from build123d import *

# Parameters (mm, degrees)
SKETCH1_R           = 1.778
BOSS_EXTRUDE1_DEPTH = 6.096
FILLET1_R           = 2.54
SKETCH2_R           = 2.4003
BOSS_EXTRUDE2_DEPTH = 13.97
CHAMFER1_SIZE       = 6.35
CHAMFER1_SIZE_2     = 0.667411894


with BuildPart() as part:
    # Sketch1 → Boss-Extrude1 (new, symmetric)
    with BuildSketch(Plane(origin=(0, 0, 0), x_dir=(1, 0, 0), z_dir=(0, 1, 0))):
        with BuildLine():
            Line((-10.16, 6.223), (-10.16, 13.716))
            Line((-10.16, 13.716), (10.16, 13.716))
            Line((10.16, 13.716), (10.16, 6.223))
            ThreePointArc((10.16, 6.223), (13.335, 3.048), (10.16, -0.127))
            Line((10.16, -0.127), (10.16, -13.716))
            Line((10.16, -13.716), (-10.16, -13.716))
            Line((-10.16, -13.716), (-10.16, -0.127))
            ThreePointArc((-10.16, -0.127), (-13.335, 3.048), (-10.16, 6.223))
        make_face()
        with Locations(Location((-10.16, 3.048, 0), (0, 0, 90))):
            Circle(SKETCH1_R, mode=Mode.SUBTRACT)
        with Locations(Location((10.16, 3.048, 0), (0, 0, 90))):
            Circle(SKETCH1_R, mode=Mode.SUBTRACT)
    extrude(amount=BOSS_EXTRUDE1_DEPTH, both=True)

    # Fillet1
    fillet1_edges = [part.edges().sort_by_distance(p)[0] for p in [
        (10.16, 0, -6.223),
        (10.16, 0, 0.127),
        (10.16, 0, 13.716),
        (-10.16, 0, 13.716),
        (-10.16, 0, 0.127),
        (-10.16, 0, -6.223),
        (-10.16, 0, -13.716),
        (10.16, 0, -13.716),
    ]]
    fillet(fillet1_edges, radius=FILLET1_R)

    # Sketch2 → Boss-Extrude2 (add)
    with BuildSketch(Plane(origin=(0, 6.096, 0), x_dir=(1, 0, 0), z_dir=(0, 1, 0))):
        with Locations(Location((0, 8.382, 0), (0, 0, 270))):
            Circle(SKETCH2_R)
        with Locations(Location((0, -2.286, 0), (0, 0, 270))):
            Circle(SKETCH2_R)
    extrude(amount=BOSS_EXTRUDE2_DEPTH)

    # Chamfer1
    # the kernel refuses this chamfer: 6.35, 0.667411894 mm, written as the material it adds along each edge
    with BuildSketch(Plane(origin=(0, 6.096, -8.382), x_dir=(0, 0, 1), z_dir=(-1, 0, 0))) as chamfer1_piece_1_section:
        Polygon((2.4003 + CHAMFER1_SIZE, 0), (2.4003, CHAMFER1_SIZE_2), (2.4003, 0), align=None)
    chamfer1_piece_1 = revolve(axis=Axis((0, 6.096, -8.382), (0, 1, 0)), mode=Mode.PRIVATE)
    chamfer1_piece_1 = split(chamfer1_piece_1, bisect_by=Plane(origin=(6.803322578, 6.146034246, -13.716), z_dir=(0, 0, 1)), keep=Keep.TOP, mode=Mode.PRIVATE)
    add(chamfer1_piece_1)
    with BuildSketch(Plane(origin=(0, 6.096, 2.286), x_dir=(0, 0, 1), z_dir=(-1, 0, 0))) as chamfer1_piece_2:
        Polygon((2.4003 + CHAMFER1_SIZE, 0), (2.4003, CHAMFER1_SIZE_2), (2.4003, 0), align=None)
    revolve(axis=Axis((0, 6.096, 2.286), (0, 1, 0)))
    # the kernel refuses this chamfer: 6.35, 0.667411894 mm, written as the material it takes off along each edge
    with BuildSketch(Plane(origin=(0, 20.066, -8.382), x_dir=(0, 0, 1), z_dir=(-1, 0, 0))) as chamfer1_2_piece_1:
        Polygon((2.4003, -CHAMFER1_SIZE), (2.4003 - CHAMFER1_SIZE_2, 0), (2.4003, 0), align=None)
    revolve(axis=Axis((0, 20.066, -8.382), (0, 1, 0)), mode=Mode.SUBTRACT)
    with BuildSketch(Plane(origin=(0, 20.066, 2.286), x_dir=(0, 0, 1), z_dir=(-1, 0, 0))) as chamfer1_2_piece_2:
        Polygon((2.4003, -CHAMFER1_SIZE), (2.4003 - CHAMFER1_SIZE_2, 0), (2.4003, 0), align=None)
    revolve(axis=Axis((0, 20.066, 2.286), (0, 1, 0)), mode=Mode.SUBTRACT)


solid = part.part
Work out the finished part from the listing and answer in its coordinate system (mm). A direction names the side the tool comes from. Give positions to 0.01 mm unless a question says otherwise; leave off trailing zeros. Order: outer loops, then holes, each group sorted by start corner. A loop starts at its lowest first (then second) coordinate and runs counter-clockwise, first axis right, second up. Notation, with made-up numbers: (70, 85.25) -> (99, 85.25) arc R33 cw to (99, 123.25) -> close; hole circle Ø2 at (75.5, 16). An arc over 180 degrees is marked (long way). One line per item, written item: value.
Item 1: Find section C-C, the plane x = 0. Give the vertices of the cut face in (y, z), plus the area to 3 significant figures.
Answer sheet:
outline: (-6.1, -13.72) -> (6.46, -13.72) -> (6.76, -10.78) -> (13.72, -10.78) -> (20.07, -10.11) -> (20.07, -6.65) -> (13.72, -5.98) -> (6.76, -5.98) -> (6.46, -3.05) -> (6.76, -0.11) -> (13.72, -0.11) -> (20.07, 0.55) -> (20.07, 4.02) -> (13.72, 4.69) -> (6.76, 4.69) -> (6.1, 11.04) -> (6.1, 13.72) -> (-6.1, 13.72) -> close
area: 467 mm²
Item 2: Find section D-D, the plane y = 7.5. Give the vertices of the cut face in (x, z), plus the area to 3 significant figures.
Answer sheet:
outline: circle Ø4.8 at (0, -8.38); circle Ø4.8 at (0, 2.29)
area: 36.2 mm²
Item 3: Find section A-A, the plane y = -0.75. Give the vertices of the cut face in (x, z) (3 decimals).
Answer sheet:
outline: (-11.571, -5.892) arc R2.54 cw to (-10.16, -8.168) -> (-10.16, -11.176) arc R2.54 ccw to (-7.62, -13.716) -> (7.62, -13.716) arc R2.54 ccw to (10.16, -11.176) -> (10.16, -8.168) arc R2.54 cw to (11.571, -5.892) arc R3.175 ccw to (11.571, -0.204) arc R2.54 cw to (10.16, 2.072) -> (10.16, 11.176) arc R2.54 ccw to (7.62, 13.716) -> (-7.62, 13.716) arc R2.54 ccw to (-10.16, 11.176) -> (-10.16, 2.072) arc R2.54 cw to (-11.571, -0.204) arc R3.175 ccw to start; hole circle Ø3.556 at (-10.16, -3.048); hole circle Ø3.556 at (10.16, -3.048)
Item 4: Straight lines are drawn through the part: probe 1 along X at (y, z) = (5, -2); probe 2 along X at (y, z) = (-1.75, 4.5); probe 3 along Z at (x, y) = (-1.5, 12). For each, find the intervals that lie inside material, in ascending order.
Answer sheet:
probe 1: -13.16 to -11.6, -8.72 to 8.72, 11.6 to 13.16
probe 2: -10.16 to 10.16
probe 3: -10.26 to -6.51, 0.41 to 4.16
Item 5: Find section B-B, the plane x = -9.75. Give the vertices of the cut face in (y, z), plus the area to 3 significant figures.
Answer sheet:
outline: (-6.1, -12.56) -> (6.1, -12.56) -> (6.1, -4.78) -> (-6.1, -4.78) -> close; (-6.1, -1.32) -> (6.1, -1.32) -> (6.1, 12.56) -> (-6.1, 12.56) -> close
area: 264 mm²
Item 6: A tool of negligible diameter and unlimited length cuts with its end or side. For faces 1 (the flat face through (10.16, 0, 7)), 2 (the cylindrical face through (0.721, 10.191, 4.575)), 3 (the flat face through (0, 0, -13.716)), from which of +Z, -Z, +X, -X, +Y, -Y can it reach the whole face along a straight path? Write none if from no direction.
Answer sheet:
face 1: +Z, +X, +Y, -Y
face 2: +Y
face 3: -Z, +X, -X, +Y, -Y
Item 7: Determine the mould class of faces 4 (the cylindrical face through (0.11, 10.19, -10.78)), 5 (the conical face through (-0.79, 16.94, -6.48)), 6 (the cylindrical face through (-13.335, 0.085, -2.999)), 7 (the flat face through (-10.16, 0, 7)) for opening direction Z: released by +Z, released by -Z, zero draft, split by the parting line, or undercut.
Answer sheet:
face 4: undercut
face 5: undercut
face 6: split by the parting line
face 7: zero draft
Item 8: Flat-ended cylindrical pins translate along their axes: P1, Ø10, axis at y = -2, z = 5.5, coming from the +X side; P2, Ø3, axis at x = -5, y = 15.5, coming from the -Z side; P3, Ø7.5, axis at y = 2, z = 5.5, coming from the -X side; P4, Ø5, axis at x = 4, y = 9.5, coming from the +Z side. Find the tip coordinate at first contact, or state that the pin passes through.
Answer sheet:
P1: x = 10.7
P2: through
P3: x = -10.18
P4: z = 4.16
